The listing builds one solid part. Answer for the finished solid, in the listing's coordinates (mm). A direction names the side the tool comes from. Give positions to 0.01 mm unless a question says otherwise; leave off trailing zeros. Loops run counter-clockwise (first coordinate to the right, second up) from the corner with the lowest first, then second, coordinate; pieces in that order, holes last.
Item 1: Section B-B, the plane z = 28 is taken. Give the vertices of the cut face in (x, y) (3 decimals), and give its area (3 significant figures).
Item 2: A tool of negligible diameter and unlimited length cuts with its end or side. For faces 1 (the face through (-440, 3.175, 21)), 2 (the face through (-579.483, 1.61, 24.112)), from which of +Z, -Z, +X, -X, +Y, -Y can it reach the whole face along a straight path? Write none if from no direction.
Item 3: Section A-A, the plane x = -395 is taken. Give the vertices of the cut face in (y, z) (3 decimals), and give its area (3 significant figures).
Item 4: The mould has two halves that part along X. Classify faces 3 (the face through (-295.914, 1.61, 24.507)), 4 (the face through (-579.483, 36.535, 24.112)), 5 (the face through (-370.823, 36.49, 17.602)), 6 (the face through (-440, 0, 12)): pulls with the +X half, pulls with the -X half, needs draft (parallel to the pull), parting line crosses it, or undercut.
Item 5: Each of these flat-tipped pins is pushed along its axis until it touches: pin 1 Ø8.5 at (x, z) = (-367.65, 17.46) entering from -Y; pin 2 Ø10 at (x, y) = (-477.5, 20) entering from +Z (3 decimals). Where does it stop, or does it pass through?
Item 6: Consider line 1 along Y through (x, z) = (-359, 28.5) (3 decimals); line 2 along X through (y, z) = (36.5, 16); line 3 along Z through (x, y) = (-301.5, 20.5) (3 decimals). Determine where each line is inside the solid, lowest interval first.
Item 7: Section C-C, the plane y = 18.5 is taken. Give the vertices of the cut face in (x, z) (3 decimals).
from build123d import *

# Parameters (mm, degrees)
SKETCH1_W           = 50.8
SKETCH1_H           = 38.1
SKETCH1_W_2         = 196.85
BOSS_EXTRUDE1_DEPTH = 31.75
SKETCH2_W           = 28.575
SKETCH2_H           = 31.75
CUT_EXTRUDE1_DEPTH  = 299.45
SKETCH3_R           = 6.35
CUT_EXTRUDE2_DEPTH  = 39.1
FILLET1_R           = 25.4
SKETCH4_R           = 3.175
CUT_EXTRUDE3_DEPTH  = 39.1
FILLET2_R           = 2


with BuildPart() as part:
    # Sketch1 → Boss-Extrude1 (new body)
    with BuildSketch(Plane.XY):
        with Locations((-561.325887252, 19.05)):
            Rectangle(SKETCH1_W, SKETCH1_H)
        with Locations((-437.500887252, 19.05)):
            Rectangle(SKETCH1_W_2, SKETCH1_H)
        with Locations((-313.675887252, 19.05)):
            Rectangle(SKETCH1_W, SKETCH1_H)
    extrude(amount=BOSS_EXTRUDE1_DEPTH)

    # Sketch2 → Cut-Extrude1 (cut, through all)
    with BuildSketch(Plane.ZY.offset(586.725887252)):
        with Locations((17.4625, 19.05)):
            Rectangle(SKETCH2_W, SKETCH2_H)
    extrude(amount=-CUT_EXTRUDE1_DEPTH, mode=Mode.SUBTRACT)

    # Sketch3 → Cut-Extrude2 (cut, through all)
    with BuildSketch(Plane.XZ):
        with Locations((-561.325887252, 12.7)):
            Circle(SKETCH3_R)
        with Locations((-313.675887252, 12.7)):
            Circle(SKETCH3_R)
    extrude(amount=-CUT_EXTRUDE2_DEPTH, mode=Mode.SUBTRACT)

    # Fillet1
    fillet1_edges = [part.edges().sort_by_distance(p)[0] for p in [
        (-586.725887252, 36.5125, 31.75),
        (-288.275887252, 1.5875, 31.75),
        (-288.275887252, 36.5125, 31.75),
        (-586.725887252, 1.5875, 31.75),
    ]]
    fillet(fillet1_edges, radius=FILLET1_R)

    # Sketch4 → Cut-Extrude3 (cut, through all)
    with BuildSketch(Plane.XZ):
        with Locations((-507.350887252, 17.4625)):
            Circle(SKETCH4_R)
        with Locations((-437.500887252, 17.4625)):
            Circle(SKETCH4_R)
        with Locations((-367.650887252, 17.4625)):
            Circle(SKETCH4_R)
    extrude(amount=-CUT_EXTRUDE3_DEPTH, mode=Mode.SUBTRACT)

    # Fillet2
    fillet2_edges = [part.edges().sort_by_distance(p)[0] for p in [
        (-437.500887252, 3.175, 3.175),
        (-437.500887252, 34.925, 3.175),
    ]]
    fillet(fillet2_edges, radius=FILLET2_R)


solid = part.part
Worked answers:
1. outline: (-574.609, 0) - (-300.393, 0) - (-300.393, 3.175) - (-574.609, 3.175) - close; (-574.609, 34.925) - (-300.393, 34.925) - (-300.393, 38.1) - (-574.609, 38.1) - close
1. area: 1,740 mm2
2. face 1: +Z, +X, -X
2. face 2: +Z, -X, +Y, -Y
3. outline: (0, 0) - (38.1, 0) - (38.1, 31.75) - (34.925, 31.75) - (34.925, 5.175) arc R2 cw to (32.925, 3.175) - (5.175, 3.175) arc R2 cw to (3.175, 5.175) - (3.175, 31.75) - (0, 31.75) - close
3. area: 304 mm2
4. face 3: pulls with the +X half
4. face 4: pulls with the -X half
4. face 5: undercut
4. face 6: needs draft
5. pin 1: stops at y = 0
5. pin 2: stops at z = 3.175
6. line 1: y = 0 to 3.175, 34.925 to 38.1
6. line 2: x = -584.82 to -566.75, -555.9 to -510.17, -504.53 to -440.32, -434.68 to -370.47, -364.83 to -319.1, -308.25 to -290.18
6. line 3: z = 0 to 3.175
7. outline: (-586.726, 0) - (-288.276, 0) - (-288.276, 3.175) - (-586.726, 3.175) - close
